Source: three-view drawing plus pictorial views. Frame: mm from the lowest corner of the part. Give positions to 0.01 mm unless a question says otherwise; leave off trailing zeros. Order: outer loops, then holes, each group sorted by start corner. A loop starts at its lowest first (then second) coordinate and runs counter-clockwise, first axis right, second up. Notation, with made-up numbers: M 30.25,70 L 74.25,70 A11 ccw 74.25,84 Z; hole C 78.25,-17 d2. An arc over 180 degrees is marked long. Use CSV: the item, a comma, the result in double quotes. Start each with the question number.
1. Section query B-B, the plane z = 67.5. Return the cut outline in (x, y).
2. Section query C-C, the plane y = 3.1. Return the cut outline in (x, z).
3. Pin query (flat end, axial travel): P1, Ø4, axis at x = 195, z = 5, coming from the +Y side. Return the tip coordinate at first contact, or that it passes through.
4. Line query: line 1 along X through (y, z) = (3.15, 95); line 2 along Z through (x, y) = (195, 3.4); line 3 along X through (y, z) = (2.55, 14.5). Output: solid intervals per line, ascending. Write a range as [from, to].
5. Section query A-A, the plane x = 66.5. Return the cut outline in (y, z), plus the area to 3 significant figures.
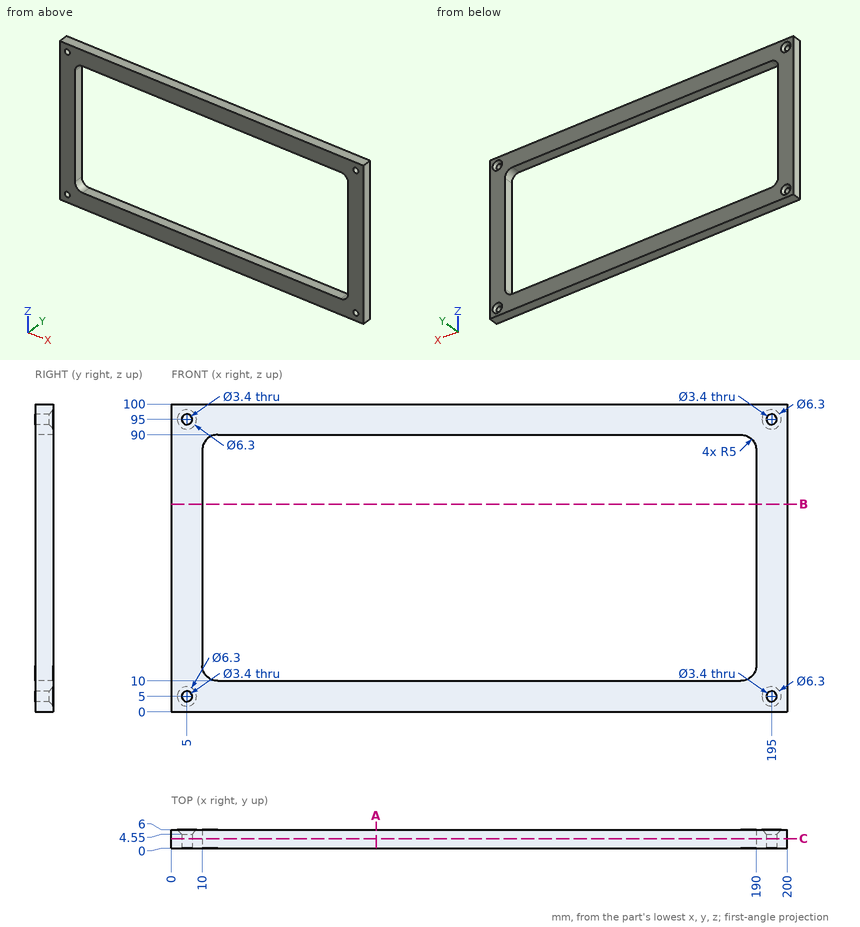
Result set:
1,outline,"M 0,0 L 10,0 L 10,6 L 0,6 Z; M 190,0 L 200,0 L 200,6 L 190,6 Z"
2,outline,"M 0,0 L 200,0 L 200,100 L 0,100 Z; hole C 5,5 d3.4; hole C 5,95 d3.4; hole M 10,15 A5 ccw 15,10 L 185,10 A5 ccw 190,15 L 190,85 A5 ccw 185,90 L 15,90 A5 ccw 10,85 Z; hole C 195,5 d3.4; hole C 195,95 d3.4"
3,P1,"y = 4.85"
4,line 1,"[0, 3.3], [6.7, 193.3], [196.7, 200]"
4,line 2,"[0, 3.3], [6.7, 93.3], [96.7, 100]"
4,line 3,"[0, 10.03], [189.97, 200]"
5,outline,"M 0,0 L 6,0 L 6,10 L 0,10 Z; M 0,90 L 6,90 L 6,100 L 0,100 Z"
5,area,"120 mm2"
